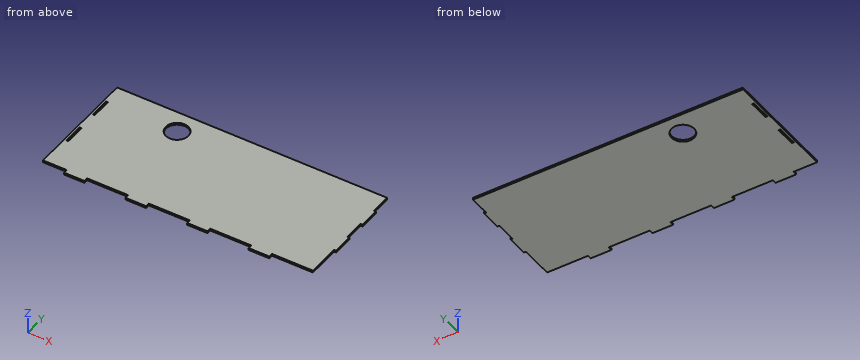
from build123d import *

# Parameters (mm, degrees)
SKETCH1_R           = 11
BOSS_EXTRUDE1_DEPTH = 2
SKETCH2_W           = 2
SKETCH2_H           = 20
CUT_EXTRUDE1_DEPTH  = 10


with BuildPart() as part:
    # Sketch1 → Boss-Extrude1 (new body)
    with BuildSketch(Plane.XY):
        Polygon((11.5, -56), (11.5, -60), (31.5, -60), (31.5, -56), (71.5, -56), (71.5, -60), (91.5, -60), (91.5, -56), (131.5, -56), (131.5, -24), (133.5, -24), (133.5, -4), (131.5, -4), (131.5, 16), (133.5, 16), (133.5, 36), (131.5, 36), (131.5, 56), (-131.5, 56), (-131.5, 36), (-131.5, 16), (-131.5, -4), (-131.5, -24), (-131.5, -56), (-108.5, -56), (-108.5, -60), (-88.5, -60), (-88.5, -56), (-48.5, -56), (-48.5, -60), (-28.5, -60), (-28.5, -56), align=None)
        with Locations((-59.5, 35)):
            Circle(SKETCH1_R, mode=Mode.SUBTRACT)
    extrude(amount=BOSS_EXTRUDE1_DEPTH)

    # Sketch2 → Cut-Extrude1 (cut)
    with BuildSketch(Plane.XY.offset(2)):
        with Locations((-128.5, 26)):
            Rectangle(SKETCH2_W, SKETCH2_H)
        with Locations((-128.5, -14)):
            Rectangle(SKETCH2_W, SKETCH2_H)
    extrude(amount=-CUT_EXTRUDE1_DEPTH, mode=Mode.SUBTRACT)


solid = part.part
The model under review builds one solid part; all positions refer to its coordinate system, in mm. Round coordinates to 2 decimals unless told otherwise and drop trailing zeros. Loops run counter-clockwise (first coordinate to the right, second up) from the corner with the lowest first, then second, coordinate; pieces in that order, holes last. Notation, with made-up numbers: M 13,87 L 25,87 A18 ccw 25,116 Z; hole C 48.5,-24 d7. An arc over 180 degrees is marked long. Answer as a JSON object with one key per item and string values.
Item 1: We need section A-A, the plane x = -59.5. State the section outline as (y, z) points.
Check sheet entries:
{"outline": "M -56,0 L 24,0 L 24,2 L -56,2 Z; M 46,0 L 56,0 L 56,2 L 46,2 Z"}
Item 2: For line 1 along X through (y, z) = (-17.5, 1.75); line 2 along Y through (x, z) = (-59.5, 0.8); line 3 along X through (y, z) = (31, 1.1), list the stretches that pass through material, from the lowest coordinate up.
Check sheet entries:
{"line 1": "-131.5 to -129.5, -127.5 to 133.5", "line 2": "-56 to 24, 46 to 56", "line 3": "-131.5 to -129.5, -127.5 to -69.75, -49.25 to 133.5"}
Item 3: We need section B-B, the plane z = 0.4. State how many separate pieces and enclosed holes the cut face has, and give its area (3 significant figures).
Check sheet entries:
{"separate pieces": "1", "enclosed holes": "3", "area": "29,400 mm2"}
Item 4: Clearance check with flat-ended pins moving along their axes: P1, Ø1, axis at x = -129, z = 1, coming from the -Y side; P2, Ø1, axis at y = 8, z = 0.5, coming from the +X side; P3, Ø1, axis at x = 132.5, z = 0.5, coming from the -Y side. State where each tip first meets the part, or that it passes through.
Check sheet entries:
{"P1": "y = -56", "P2": "x = 131.5", "P3": "y = -24"}
